Here's how the part is built. I have some questions about the finished solid (model axes, mm). Coordinates: 2 decimals unless noted, no trailing zeros. Write each loop counter-clockwise with the first axis right and the second up, starting at its lowest first coordinate (ties: lowest second). Pieces come first, ordered by that corner, then holes. Notation, with made-up numbers: (58, -28) -> (83, -28) arc R20 ccw to (83, -16) -> close; hole circle Ø1 at (-19, 11.5). An arc over 180 degrees is marked (long way). Put each result on its own line as item: value. Start each with the question number.
Item 1: I want a section at A-A, the plane x = 11.5. List the corners of the cut face in (y, z) for me.
Item 2: For pin 1 (2 mm diameter, centred on y = 66, z = 3, fed in from +X); pin 2 (3 mm diameter, centred on y = 84.5, z = 3, fed in from -X); pin 3 (1.8 mm diameter, centred on x = 68.5, z = 4, fed in from -Y), each with a flat end and sliding along its axis, tell me the tip position at first contact or that it passes through.
Item 3: I need wall thicknesses on line 1 (X direction, y = 131, z = 3.9); line 2 (X direction, y = 54, z = 2.85). Which ranges of each line are inside material? Lowest first, please. Write a range as [from, to].
Item 4: I want a section at D-D, the plane x = 61.5. List the corners of the cut face in (y, z) for me.
Item 5: I want a section at C-C, the plane z = 2.05. List the corners of the cut face in (x, y) for me.
Autodesk Inventor part; units mm, degrees
ref_plane "YZ Plane" through (0, 0, 0) normal (1, 0, 0) x (0, 1, 0)
ref_plane "XZ Plane" through (0, 0, 0) normal (0, 1, 0) x (-1, 0, 0)
ref_plane "XY Plane" through (0, 0, 0) normal (0, 0, 1) x (1, 0, 0)
sketch "Szkic1" plane through (0, 0, 0) normal (0, 0, 1) x (1, 0, 0)
  line L0 (0, 0) -> (152, 0) construction
  line L1 (152, 0) -> (152, 152) construction
  line L2 (152, 152) -> (0, 152) construction
  line L3 (0, 152) -> (0, 0) construction
  line L4 (129.5, 22.5) -> (22.5, 22.5) construction
  line L5 (22.5, 22.5) -> (22.5, 129.5) construction
  line L6 (22.5, 129.5) -> (129.5, 129.5) construction
  line L7 (129.5, 129.5) -> (129.5, 22.5) construction
  line L8 (0, 0) -> (45, 0) construction
  line L9 (45, 0) -> (45, 45) construction
  line L10 (45, 45) -> (0, 45) construction
  line L11 (0, 45) -> (0, 0) construction
  line L12 (0, 152) -> (45, 152) construction
  line L13 (45, 152) -> (45, 107) construction
  line L14 (45, 107) -> (0, 107) construction
  line L15 (0, 107) -> (0, 152) construction
  line L16 (152, 152) -> (107, 152) construction
  line L17 (107, 152) -> (107, 107) construction
  line L18 (107, 107) -> (152, 107) construction
  line L19 (152, 107) -> (152, 152) construction
  line L20 (152, 0) -> (107, 0) construction
  line L21 (107, 0) -> (107, 45) construction
  line L22 (107, 45) -> (152, 45) construction
  line L23 (152, 45) -> (152, 0) construction
  line L24 (0, 0) -> (45, 0)
  line L25 (45, 0) -> (45, 22.5)
  line L26 (45, 22.5) -> (107, 22.5)
  line L27 (107, 22.5) -> (107, 0)
  line L28 (107, 0) -> (152, 0)
  line L29 (152, 0) -> (152, 45)
  line L30 (152, 45) -> (129.5, 45)
  line L31 (129.5, 45) -> (129.5, 107)
  line L32 (129.5, 107) -> (152, 107)
  line L33 (152, 107) -> (152, 152)
  line L34 (152, 152) -> (107, 152)
  line L35 (107, 152) -> (107, 129.5)
  line L36 (107, 129.5) -> (45, 129.5)
  line L37 (45, 129.5) -> (45, 152)
  line L38 (45, 152) -> (0, 152)
  line L39 (0, 152) -> (0, 107)
  line L40 (0, 107) -> (22.5, 107)
  line L41 (22.5, 107) -> (22.5, 45)
  line L42 (22.5, 45) -> (0, 45)
  line L43 (0, 45) -> (0, 0)
  dimension "d0" = 152
  dimension "d1" = 152
  dimension "d2" = 22.5
  dimension "d3" = 45
  dimension "d4" = 45
  dimension "d5" = 45
  dimension "d6" = 45
  dimension "d7" = 45
  dimension "d8" = 45
  dimension "d9" = 45
  dimension "d10" = 45
extrude "Wyciągnięcie proste1" add sketch "Szkic1" along normal blind 6
equation "\"d1\" = d0"
properties part number "Pokrywka"
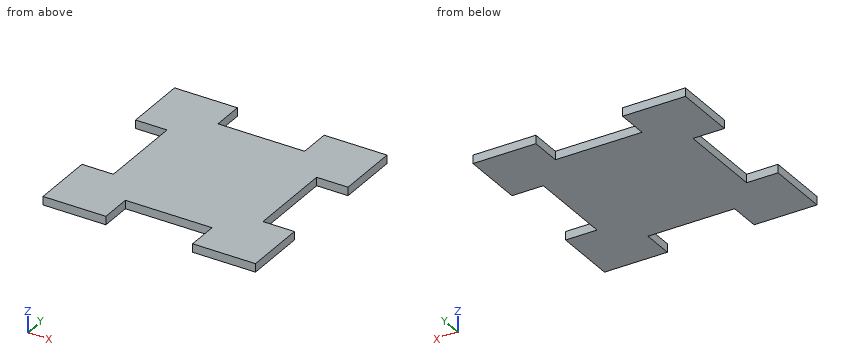
Calculated:
1. outline: (0, 0) -> (45, 0) -> (45, 6) -> (0, 6) -> close; (107, 0) -> (152, 0) -> (152, 6) -> (107, 6) -> close
2. pin 1: stops at x = 129.5
2. pin 2: stops at x = 22.5
2. pin 3: stops at y = 22.5
3. line 1: x = [0, 45], [107, 152]
3. line 2: x = [22.5, 129.5]
4. outline: (22.5, 0) -> (129.5, 0) -> (129.5, 6) -> (22.5, 6) -> close
5. outline: (0, 0) -> (45, 0) -> (45, 22.5) -> (107, 22.5) -> (107, 0) -> (152, 0) -> (152, 45) -> (129.5, 45) -> (129.5, 107) -> (152, 107) -> (152, 152) -> (107, 152) -> (107, 129.5) -> (45, 129.5) -> (45, 152) -> (0, 152) -> (0, 107) -> (22.5, 107) -> (22.5, 45) -> (0, 45) -> close
